from build123d import *

# Parameters (mm, degrees)
CHAMFER1_SIZE = 0.3


with BuildPart() as part:
    # Sketch1 → Revolve1 (revolve)
    with BuildSketch(Plane.XY):
        Polygon((-6.79253012, 1.45), (-1.79253012, 1.45), (-1.79253012, 1.5), (3.20746988, 1.5), (3.20746988, 0), (-6.79253012, 0), align=None)
    revolve(axis=Axis((-2.508674699, 0, 0), (1, 0, 0)))

    # Chamfer1
    chamfer1_edges = [part.edges().sort_by_distance(p)[0] for p in [
        (3.20746988, -1.5, 0),
        (-6.79253012, -1.45, 0),
    ]]
    chamfer(chamfer1_edges, length=CHAMFER1_SIZE)


solid = part.part
Here's how the part is built. I have some questions about the finished solid (model axes, mm). A direction names the side the tool comes from. Round coordinates to 2 decimals unless told otherwise and drop trailing zeros. Order: outer loops, then holes, each group sorted by start corner. A loop starts at its lowest first (then second) coordinate and runs counter-clockwise, first axis right, second up. Notation, with made-up numbers: M 37,59.25 L 52,59.25 A14 cw 52,69.25 Z; hole C 5.5,7 d9. An arc over 180 degrees is marked long. One line per question, with ' | ' between items.
1) Imagine slicing it at D-D, the plane x = -5. Write out the boundary of the cut face in (y, z).
Checked values:
outline: C 0,0 d2.9
2) I need wall thicknesses on line 1 (Z direction, x = 0, y = -0.9); line 2 (X direction, y = -1.25, z = 0.25); line 3 (Z direction, x = 2.25, y = 1). Which ranges of each line are inside material? Lowest first, please.
Checked values:
line 1: z = -1.2 to 1.2 | line 2: x = -6.67 to 3.13 | line 3: z = -1.12 to 1.12
3) Imagine slicing it at A-A, the plane y = 0. Write out the boundary of the cut face in (x, z), plus the area to 3 significant figures.
Checked values:
outline: M -6.79,-1.15 L -6.49,-1.45 L -1.79,-1.45 L -1.79,-1.5 L 2.91,-1.5 L 3.21,-1.2 L 3.21,1.2 L 2.91,1.5 L -1.79,1.5 L -1.79,1.45 L -6.49,1.45 L -6.79,1.15 Z | area: 29.3 mm²
4) Imagine slicing it at C-C, the plane x = 1.75. Write out the boundary of the cut face in (y, z), plus the area to 3 significant figures.
Checked values:
outline: C 0,0 d3 | area: 7.07 mm²
5) On a 3-axis mill with a long thin cutter (end or side, diameter ignored), from which of +Z, -Z, +X, -X, +Y, -Y can I reach the whole of each face in a straight line? I mean faces 1 (the cylindrical face through (-4.11, -1.45, 0.06)), 2 (the flat face through (-6.793, 0, 0)). Say none if no direction works.
Checked values:
face 1: -X | face 2: +Z, -Z, -X, +Y, -Y
6) I'm going to push a flat-ended pin straight in: pin 1 Ø1.5 at (y, z) = (-1, -1) entering from -X. Where does the tip first touch, or does it pass through?
Checked values:
pin 1: stops at x = -6.79
